Autodesk Inventor part; units mm, degrees
ref_plane "YZ Plane" through (0, 0, 0) normal (1, 0, 0) x (0, 1, 0)
ref_plane "XZ Plane" through (0, 0, 0) normal (0, 1, 0) x (-1, 0, 0)
ref_plane "XY Plane" through (0, 0, 0) normal (0, 0, 1) x (1, 0, 0)
sketch "Sketch1" plane through (0, 0, 0) normal (0, 0, 1) x (1, 0, 0)
  line L0 (0, 0) -> (25.4, 0)
  line L1 (25.4, 0) -> (25.4, 25.4)
  line L2 (25.4, 25.4) -> (0, 25.4)
  line L3 (0, 25.4) -> (0, 0)
  line L4 (3.175, 22.225) -> (22.225, 22.225)
  line L5 (22.225, 22.225) -> (22.225, 3.175)
  line L6 (22.225, 3.175) -> (3.175, 3.175)
  line L7 (3.175, 3.175) -> (3.175, 22.225)
  dimension "d0" = 25.4
  dimension "d1" = 25.4
  dimension "d2" = 3.175
extrude "Extrusion1" add sketch "Sketch1" along normal blind 101.6
sketch "Sketch2" plane through (0, 25.4, 0) normal (0, 1, 0) x (1, 0, 0)
  line L0 (0, 0) -> (25.4, 0) construction
  line L1 (12.7, 0) -> (12.7, -12.7) construction
  line L2 (12.7, -12.7) -> (12.7, -38.1) construction
  line L3 (12.7, -38.1) -> (12.7, -63.5) construction
  line L4 (12.7, -63.5) -> (12.7, -88.9) construction
  circle A0 centre (12.7, -88.9) radius 2.5797
  circle A1 centre (12.7, -63.5) radius 2.5797
  circle A2 centre (12.7, -38.1) radius 2.5797
  circle A3 centre (12.7, -12.7) radius 2.5797
  dimension "d5" = 12.7
  dimension "d6" = 25.4
  dimension "d7" = 25.4
  dimension "d8" = 25.4
  dimension "d9" = 5.1594
extrude "Extrusion2" cut sketch "Sketch2" against normal blind 101.6
properties part number "4in 1x1"
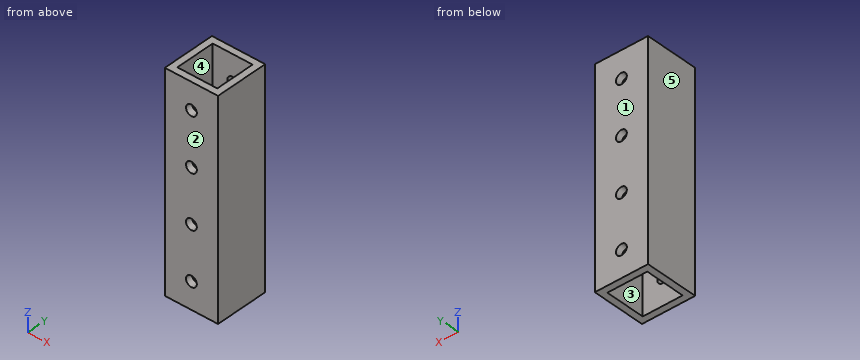
Verification items for the finished model (mm, model axes). Face numbers are marked on the shaded views. A direction names the side the tool comes from. Round coordinates to 2 decimals unless told otherwise and drop trailing zeros. Order: outer loops, then holes, each group sorted by start corner. A loop starts at its lowest first (then second) coordinate and runs counter-clockwise, first axis right, second up.
1. Access from +Z, -Z, +X, -X, +Y, -Y to the whole of each face (thin tool, end or side, straight path). Record for the marked faces 4 and 5.
Final values:
face 4: +Z, -Z
face 5: +Z, -Z, -X, +Y, -Y
2. Go/stop test with a flat-tipped pin: P1, Ø3, axis at x = 12.7, z = 38.1, coming from the +Y side. Record where the tip stops, or that it passes through.
Final values:
P1: passes through
3. Thickness scan on L1, parallel to Z at x = 12.7, y = 23.95; L2, parallel to X at y = 1.7, z = 12.7; L3, parallel to Y at x = 10, z = 34 (3 decimals). Record the ranges inside material, lowest first.
Final values:
L1: z = 0 to 10.12, 15.28 to 35.52, 40.68 to 60.92, 66.08 to 86.32, 91.48 to 101.6
L2: x = 0 to 10.12, 15.28 to 25.4
L3: y = 0 to 3.175, 22.225 to 25.4
4. Section check A-A on x = 7. Record the cut outline in (y, z) (3 decimals), then the cut area to 3 significant figures.
Final values:
outline: (0, 0) - (3.175, 0) - (3.175, 101.6) - (0, 101.6) - close; (22.225, 0) - (25.4, 0) - (25.4, 101.6) - (22.225, 101.6) - close
area: 645 mm2
5. Section check D-D on z = 80.5. Record the cut outline in (x, y) (3 decimals), then the cut area to 3 significant figures.
Final values:
outline: (0, 0) - (25.4, 0) - (25.4, 25.4) - (0, 25.4) - close; hole (3.175, 3.175) - (22.225, 3.175) - (22.225, 22.225) - (3.175, 22.225) - close
area: 282 mm2
6. Release check for a two-part mould opening along Y. For the marked faces 1, 2 and 3 record: +Y half, -Y half, draft (parallel to the pull), parting line (faces both ways), or undercut.
Final values:
face 1: +Y half
face 2: -Y half
face 3: undercut
7. Section check C-C on z = 63.5. Record the cut outline in (x, y) (3 decimals).
Final values:
outline: (0, 0) - (10.12, 0) - (10.12, 3.175) - (3.175, 3.175) - (3.175, 22.225) - (10.12, 22.225) - (10.12, 25.4) - (0, 25.4) - close; (15.28, 0) - (25.4, 0) - (25.4, 25.4) - (15.28, 25.4) - (15.28, 22.225) - (22.225, 22.225) - (22.225, 3.175) - (15.28, 3.175) - close
